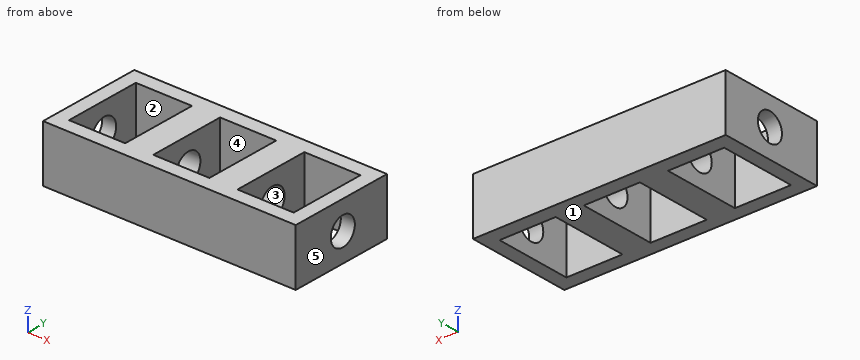
from build123d import *

# Parameters (mm, degrees)
SKETCH_W        = 180
SKETCH_H        = 75.807773
PAD_DEPTH       = 40
SKETCH001_W     = 40
SKETCH001_H     = 55.5
POCKET_DEPTH    = 40
SKETCH002_R     = 10.002665
POCKET001_DEPTH = 257


with BuildPart() as part:
    # Sketch → Pad (new body)
    with BuildSketch(Plane.XY):
        with Locations((90, -37.903886)):
            Rectangle(SKETCH_W, SKETCH_H)
    extrude(amount=PAD_DEPTH)

    # Sketch001 (on Face6 of Pad) → Pocket (cut)
    with BuildSketch(Plane.XY.offset(40)):
        with Locations((30, -38.113381)):
            Rectangle(SKETCH001_W, SKETCH001_H)
        with Locations((90, -38.113381)):
            Rectangle(SKETCH001_W, SKETCH001_H)
        with Locations((150, -38.113381)):
            Rectangle(SKETCH001_W, SKETCH001_H)
    extrude(amount=-POCKET_DEPTH, mode=Mode.SUBTRACT)

    # Sketch002 (on Face2 of Pocket) → Pocket001 (cut)
    with BuildSketch(Plane(origin=(0, 0, 0), x_dir=(0, -1, 0), z_dir=(-1, 0, 0))):
        with Locations((36.707787, 20)):
            Circle(SKETCH002_R)
    extrude(amount=-POCKET001_DEPTH, mode=Mode.SUBTRACT)


solid = part.part
Input: part model. Units: mm. Frame: model coordinates. Face numbers are marked on the shaded views. A direction names the side the tool comes from. Give positions to 0.01 mm unless a question says otherwise; leave off trailing zeros. Loops run counter-clockwise (first coordinate to the right, second up) from the corner with the lowest first, then second, coordinate; pieces in that order, holes last. Notation, with made-up numbers: M 4,-24.75 L 43,-24.75 A9 ccw 43,-11.75 Z; hole C -40,8 d10. An arc over 180 degrees is marked long. Use CSV: the item, a comma, the result in double quotes.
(1) Section C-C, the plane x = 39. Return loops of the section in (y, z), plus the area to 3 significant figures.
Outcome:
outline,"M -75.81,0 L -65.86,0 L -65.86,40 L -75.81,40 Z; M -10.36,0 L 0,0 L 0,40 L -10.36,40 Z"
area,"812 mm²"
(2) Material intervals for L1, parallel to X at y = -49, z = 25.5; L2, parallel to Y at x = 17.5, z = 26.5; L3, parallel to Z at x = 63, y = -40, sorted ascending. Write a range as [from, to].
Outcome:
L1,"x = [0, 10], [50, 70], [110, 130], [170, 180]"
L2,"y = [-75.81, -65.86], [-10.36, 0]"
L3,"z = [0, 10.55], [29.45, 40]"
(3) Pull-direction query (Z, two-part tool) for the marked faces 1, 2 and 3; classes: pulls with the +Z half, pulls with the -Z half, needs draft (parallel to the pull), parting line crosses it, or undercut.
Outcome:
face 1,"pulls with the -Z half"
face 2,"needs draft"
face 3,"undercut"
(4) Section A-A, the plane z = 34. Return loops of the section in (x, y).
Outcome:
outline,"M 0,-75.81 L 180,-75.81 L 180,0 L 0,0 Z; hole M 10,-65.86 L 50,-65.86 L 50,-10.36 L 10,-10.36 Z; hole M 70,-65.86 L 110,-65.86 L 110,-10.36 L 70,-10.36 Z; hole M 130,-65.86 L 170,-65.86 L 170,-10.36 L 130,-10.36 Z"
(5) Set-up query: the marked faces 4 and 5. Return all of +Z, -Z, +X, -X, +Y, -Y with unobstructed straight access to the full face (end or side cutting, diameter ignored); none if empty.
Outcome:
face 4,"+Z, -Z"
face 5,"+Z, -Z, +X, +Y, -Y"
(6) Section D-D, the plane y = -55. Return loops of the section in (x, z).
Outcome:
outline,"M 0,0 L 10,0 L 10,40 L 0,40 Z; M 50,0 L 70,0 L 70,40 L 50,40 Z; M 110,0 L 130,0 L 130,40 L 110,40 Z; M 170,0 L 180,0 L 180,40 L 170,40 Z"
